Here's how the part is built. I have some questions about the finished solid (model axes, mm). A direction names the side the tool comes from. Coordinates: 2 decimals unless noted, no trailing zeros. Write each loop counter-clockwise with the first axis right and the second up, starting at its lowest first coordinate (ties: lowest second). Pieces come first, ordered by that corner, then holes.
(1) Imagine slicing it at C-C, the plane y = 5.25. State how many separate pieces and enclosed holes the cut face has, plus the area to 3 significant figures.
(2) Imagine slicing it at B-B, the plane x = 34. List the corners of the cut face in (y, z) for me, plus the area to 3 significant figures.
(3) Imagine slicing it at D-D, the plane z = 49. List the corners of the cut face in (x, y) for me.
(4) Imagine slicing it at A-A, the plane z = 36. List the corners of the cut face in (x, y) for me.
(5) For pin 1 Ø4 at (x, z) = (18, 24) entering from +Y, with a flat end and sliding along its axis, tell me the tip position at first contact or that it passes through.
(6) Thinking about a two-plate mould opening in X: for faces 1 (the cylindrical face through (54.17, 3.94, 55.12)), 2 (the flat face through (63, 5, 0)), 3 (the flat face through (0, 5, 43)), which applies, released by +X, released by -X, zero draft, split by the parting line, or undercut?
(7) Which directions (+Z, -Z, +X, -X, +Y, -Y) give clear straight access to the entire face, cutting with the end or side of a thin tool? Please do faces 4 (the cylindrical face through (7.026, 5.356, 32.813)), 5 (the flat face through (59, 0, 40)), 6 (the flat face through (63, 8, 43)).
(8) Please list where these lines run through material, in increasing order: probe 1 along Z at (x, y) = (93.8, 0.85); probe 2 along Z at (x, y) = (34, 0.75); probe 3 along X at (y, z) = (6.5, 43.5).
```python
from build123d import *

# Parameters (mm, degrees)
SKETCH1_W           = 127.8
SKETCH1_H           = 85.8
BOSS_EXTRUDE1_DEPTH = 9.3
SKETCH2_R           = 27
CUT_EXTRUDE1_DEPTH  = 8
SKETCH3_R           = 18
CUT_EXTRUDE2_DEPTH  = 9
FILLET1_R           = 3
CUT_EXTRUDE3_DEPTH  = 8
FILLET2_R           = 2
FILLET3_R           = 3.5


with BuildPart() as part:
    # Sketch1 → Boss-Extrude1 (new body)
    with BuildSketch(Plane(origin=(0, 0, 0), x_dir=(1, 0, 0), z_dir=(0, 1, 0))):
        with Locations((63.9, -42.9)):
            Rectangle(SKETCH1_W, SKETCH1_H)
    extrude(amount=BOSS_EXTRUDE1_DEPTH)

    # Sketch2 → Cut-Extrude1 (cut)
    with BuildSketch(Plane(origin=(0, 9.3, 0), x_dir=(1, 0, 0), z_dir=(0, 1, 0))):
        with Locations((93.8, -51.8)):
            Circle(SKETCH2_R)
        with Locations((34, -34)):
            Circle(SKETCH2_R)
    extrude(amount=-CUT_EXTRUDE1_DEPTH, mode=Mode.SUBTRACT)

    # Sketch3 → Cut-Extrude2 (cut)
    with BuildSketch(Plane(origin=(0, 1.3, 0), x_dir=(1, 0, 0), z_dir=(0, 1, 0))):
        with Locations((93.8, -51.8)):
            Circle(SKETCH3_R)
        with Locations((34, -34)):
            Circle(SKETCH3_R)
    extrude(amount=-CUT_EXTRUDE2_DEPTH, mode=Mode.SUBTRACT)

    # Fillet1
    fillet1_edges = [part.edges().sort_by_distance(p)[0] for p in [
        (0, 4.65, 0),
        (127.8, 4.65, 0),
        (127.8, 4.65, 85.8),
        (0, 4.65, 85.8),
    ]]
    fillet(fillet1_edges, radius=FILLET1_R)

    # Sketch4 → Cut-Extrude3 (cut)
    with BuildSketch(Plane.XZ):
        with BuildLine():
            Line((52, 2), (124.8, 2))
            Line((124.8, 2), (125.8, 2))
            Line((125.8, 2), (125.8, 3))
            Line((125.8, 3), (125.8, 33.8))
            Line((125.8, 33.8), (116.8, 33.8))
            ThreePointArc((116.8, 33.8), (73.148123572, 31.148123572), (75.8, 74.8))
            Line((75.8, 74.8), (75.8, 83.8))
            Line((75.8, 83.8), (3, 83.8))
            Line((3, 83.8), (2, 83.8))
            Line((2, 83.8), (2, 82.8))
            Line((2, 82.8), (2, 52))
            Line((2, 52), (11, 52))
            ThreePointArc((11, 52), (54.651876428, 54.651876428), (52, 11))
            Line((52, 11), (52, 2))
        make_face()
        Polygon((125.3, 83.3), (125.3, 65.3), (121.8, 65.3), (107.3, 79.8), (107.3, 83.3), align=None)
        Polygon((2.5, 20.5), (2.5, 2.5), (20.5, 2.5), (20.5, 6), (6, 20.5), align=None)
    extrude(amount=-CUT_EXTRUDE3_DEPTH, mode=Mode.SUBTRACT)

    # Fillet2
    fillet2_edges = [part.edges().sort_by_distance(p)[0] for p in [
        (2.5, 4, 20.5),
        (6, 4, 20.5),
        (20.5, 4, 6),
        (20.5, 4, 2.5),
        (2.5, 4, 2.5),
        (121.8, 4, 65.3),
        (107.3, 4, 79.8),
        (107.3, 4, 83.3),
        (125.3, 4, 83.3),
        (125.3, 4, 65.3),
    ]]
    fillet(fillet2_edges, radius=FILLET2_R)

    # Fillet3
    fillet3_edges = [part.edges().sort_by_distance(p)[0] for p in [
        (125.8, 4, 2),
        (52, 4, 2),
        (52, 4, 11),
        (11, 4, 52),
        (2, 4, 52),
        (2, 4, 83.8),
        (75.8, 4, 83.8),
        (75.8, 4, 74.8),
        (116.8, 4, 33.8),
        (125.8, 4, 33.8),
    ]]
    fillet(fillet3_edges, radius=FILLET3_R)


solid = part.part
```
Recorded:
1. separate pieces: 1
1. enclosed holes: 5
1. area: 2,250 mm2
2. outline: (0, 0) - (9.3, 0) - (9.3, 7) - (1.3, 7) - (1.3, 16) - (0, 16) - close; (0, 52) - (1.3, 52) - (1.3, 61) - (9.3, 61) - (9.3, 85.8) - (0, 85.8) - (0, 83.8) - (8, 83.8) - (8, 63.21) - (0, 63.21) - close
2. area: 154 mm2
3. outline: (0, 0) - (24.05, 0) - (24.05, 1.3) - (11.55, 1.3) - (11.55, 9.3) - (0, 9.3) - close; (43.95, 0) - (59.06, 0) - (59.06, 8) - (64.73, 8) - (64.73, 0) - (76.02, 0) - (76.02, 1.3) - (66.95, 1.3) - (66.95, 9.3) - (56.45, 9.3) - (56.45, 1.3) - (43.95, 1.3) - close; (111.58, 0) - (127.8, 0) - (127.8, 9.3) - (120.65, 9.3) - (120.65, 1.3) - (111.58, 1.3) - close
4. outline: (0, 0) - (16.11, 0) - (16.11, 1.3) - (7.07, 1.3) - (7.07, 9.3) - (0, 9.3) - close; (51.89, 0) - (63.14, 0) - (63.14, 8) - (69.24, 8) - (69.24, 0) - (85.18, 0) - (85.18, 1.3) - (71.91, 1.3) - (71.91, 9.3) - (60.93, 9.3) - (60.93, 1.3) - (51.89, 1.3) - close; (102.42, 0) - (127.8, 0) - (127.8, 9.3) - (115.69, 9.3) - (115.69, 1.3) - (102.42, 1.3) - close
5. pin 1: stops at y = 1.3
6. face 1: undercut
6. face 2: zero draft
6. face 3: released by -X
7. face 4: +Y
7. face 5: +Z, -Z, +X, -X, -Y
7. face 6: -Y
8. probe 1: z = 0 to 2, 22.59 to 33.8, 69.8 to 85.8
8. probe 2: z = 0 to 16, 52 to 63.21, 83.8 to 85.8
8. probe 3: x = 0 to 8.73, 59.27 to 61.62, 65.8 to 68.11, 119.49 to 127.8
